Design review of the part built by this model. Coordinates are the model's own, in mm. Give positions to 0.01 mm unless a question says otherwise; leave off trailing zeros. Order: outer loops, then holes, each group sorted by start corner. A loop starts at its lowest first (then second) coordinate and runs counter-clockwise, first axis right, second up. Notation, with made-up numbers: (68.5, 43.5) -> (77.5, 43.5) arc R20 cw to (77.5, 78.5) -> close; hole circle Ø6 at (18.25, 34.25). An arc over 180 degrees is marked (long way). Use a Markdown table: item, result. Add a question column.
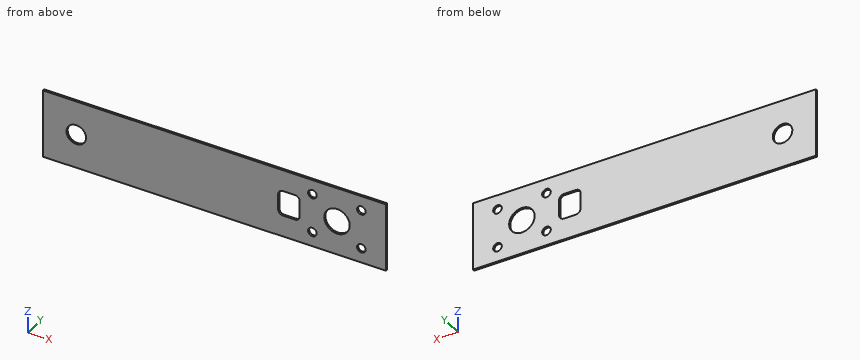
```python
from build123d import *

# Parameters (mm, degrees)
SKETCH1_W           = 350
SKETCH1_H           = 70
SKETCH1_R           = 4.4
BOSS_EXTRUDE1_DEPTH = 2
CUT_EXTRUDE1_REACH  = 180.477
SKETCH2_R           = 13
CUT_EXTRUDE2_REACH  = 180.477
SKETCH3_R           = 10


with BuildPart() as part:
    # Sketch1 → Boss-Extrude1 (new body)
    with BuildSketch(Plane(origin=(0, 0, 0), x_dir=(1, 0, 0), z_dir=(0, 1, 0))):
        Rectangle(SKETCH1_W, SKETCH1_H)
        with Locations(Location((150, 20, 0), (0, 0, 270))):
            Circle(SKETCH1_R, mode=Mode.SUBTRACT)
        with Locations(Location((150, -20, 0), (0, 0, 90))):
            Circle(SKETCH1_R, mode=Mode.SUBTRACT)
        with Locations(Location((100, -20, 0), (0, 0, 270))):
            Circle(SKETCH1_R, mode=Mode.SUBTRACT)
        with Locations(Location((100, 20, 0), (0, 0, 90))):
            Circle(SKETCH1_R, mode=Mode.SUBTRACT)
        with BuildLine():
            Line((82.1, -13), (70.1, -13))
            ThreePointArc((70.1, -13), (66.564466094, -11.535533906), (65.1, -8))
            Line((65.1, -8), (65.1, 8))
            ThreePointArc((65.1, 8), (66.564466094, 11.535533906), (70.1, 13))
            Line((70.1, 13), (82.1, 13))
            ThreePointArc((82.1, 13), (85.635533906, 11.535533906), (87.1, 8))
            Line((87.1, 8), (87.1, -8))
            ThreePointArc((87.1, -8), (85.635533906, -11.535533906), (82.1, -13))
        make_face(mode=Mode.SUBTRACT)
    extrude(amount=BOSS_EXTRUDE1_DEPTH)

    # Sketch2 → Cut-Extrude1 (cut, up to next)
    with BuildSketch(Plane(origin=(0, 0, 0), x_dir=(1, 0, 0), z_dir=(0, 1, 0)), mode=Mode.PRIVATE) as cut_extrude1_sk1:
        with Locations(Location((125.1, 0, 0), (0, 0, 90))):
            Circle(SKETCH2_R)
    cut_extrude1_tool1 = extrude(cut_extrude1_sk1.sketch, amount=CUT_EXTRUDE1_REACH, mode=Mode.PRIVATE) & part.part
    add(cut_extrude1_tool1.solids().sort_by_distance((125.1, 0, 0))[0], mode=Mode.SUBTRACT)

    # Sketch3 → Cut-Extrude2 (cut, up to next)
    with BuildSketch(Plane(origin=(0, 0, 0), x_dir=(1, 0, 0), z_dir=(0, 1, 0)), mode=Mode.PRIVATE) as cut_extrude2_sk1:
        with Locations(Location((-141, 0, 0), (0, 0, 90))):
            Circle(SKETCH3_R)
    cut_extrude2_tool1 = extrude(cut_extrude2_sk1.sketch, amount=CUT_EXTRUDE2_REACH, mode=Mode.PRIVATE) & part.part
    add(cut_extrude2_tool1.solids().sort_by_distance((-141, 0, 0))[0], mode=Mode.SUBTRACT)


solid = part.part
```
1) Add section A-A (x = 125.1). Give the boundary of the cut face in (y, z), then the cut area to 3 significant figures.
2) Add section D-D (y = 0.7). Give the boundary of the cut face in (x, z), then the cut area to 3 significant figures.
3) For L1, parallel to X at y = 1.95, z = -20; L2, parallel to Z at x = 72.5, y = 0.45; L3, parallel to X at y = 0.9, z = 0, list the stretches that pass through material, from the lowest coordinate up. Write a range as [from, to].
4) Add section C-C (z = 20). Give the boundary of the cut face in (x, y), then the cut area to 3 significant figures.
5) Add section B-B (z = 0). Give the boundary of the cut face in (x, y).
Worked answers:
| question | item | result |
|---|---|---|
| 1 | outline | (0, -35) -> (2, -35) -> (2, -13) -> (0, -13) -> close; (0, 13) -> (2, 13) -> (2, 35) -> (0, 35) -> close |
| 1 | area | 88.0 mm^2 |
| 2 | outline | (-175, -35) -> (175, -35) -> (175, 35) -> (-175, 35) -> close; hole circle Ø20 at (-141, 0); hole (65.1, -8) arc R5 ccw to (70.1, -13) -> (82.1, -13) arc R5 ccw to (87.1, -8) -> (87.1, 8) arc R5 ccw to (82.1, 13) -> (70.1, 13) arc R5 ccw to (65.1, 8) -> close; hole circle Ø8.8 at (100, -20); hole circle Ø8.8 at (100, 20); hole circle Ø26 at (125.1, 0); hole circle Ø8.8 at (150, -20); hole circle Ø8.8 at (150, 20) |
| 2 | area | 22,900 mm^2 |
| 3 | L1 | [-175, 95.6], [104.4, 145.6], [154.4, 175] |
| 3 | L2 | [-35, -13], [13, 35] |
| 3 | L3 | [-175, -151], [-131, 65.1], [87.1, 112.1], [138.1, 175] |
| 4 | outline | (-175, 0) -> (95.6, 0) -> (95.6, 2) -> (-175, 2) -> close; (104.4, 0) -> (145.6, 0) -> (145.6, 2) -> (104.4, 2) -> close; (154.4, 0) -> (175, 0) -> (175, 2) -> (154.4, 2) -> close |
| 4 | area | 665 mm^2 |
| 5 | outline | (-175, 0) -> (-151, 0) -> (-151, 2) -> (-175, 2) -> close; (-131, 0) -> (65.1, 0) -> (65.1, 2) -> (-131, 2) -> close; (87.1, 0) -> (112.1, 0) -> (112.1, 2) -> (87.1, 2) -> close; (138.1, 0) -> (175, 0) -> (175, 2) -> (138.1, 2) -> close |
